```python
from build123d import *

# Parameters (mm, degrees)
CUT_EXTRUDE_1_DEPTH = 3
FILLET_1_R          = 0.3
CHAMFER_1_SIZE      = 1


with BuildPart() as part:
    # Эскиз1 → Повернуть1 (revolve)
    with BuildSketch(Plane.XY, mode=Mode.PRIVATE) as revolve_1_sk:
        Polygon((0, 0), (0, 5.9), (0.5, 5.9), (4, 3), (16, 3), (16, 0), align=None)
    revolve(revolve_1_sk.sketch.rotate(Axis((0, 0, 0), (1, 0, 0)), 90), axis=Axis((0, 0, 0), (1, 0, 0)))  # turned: the seam where the file's is

    # Эскиз2 → Вырез-Вытянуть1 (cut)
    with BuildSketch(Plane.ZY):
        Polygon((1.154700538, 2), (-1.154700538, 2), (-2.309401077, 0), (-1.154700538, -2), (1.154700538, -2), (2.309401077, 0), align=None)
    extrude(amount=-CUT_EXTRUDE_1_DEPTH, mode=Mode.SUBTRACT)

    # Скругление1
    fillet_1_edges = [part.edges().sort_by_distance(p)[0] for p in [
        (0, 0, -5.9),
    ]]
    fillet(fillet_1_edges, radius=FILLET_1_R)

    # Фаска1
    chamfer_1_edges = [part.edges().sort_by_distance(p)[0] for p in [
        (16, 0, -3),
    ]]
    chamfer(chamfer_1_edges, length=CHAMFER_1_SIZE)


solid = part.part
```
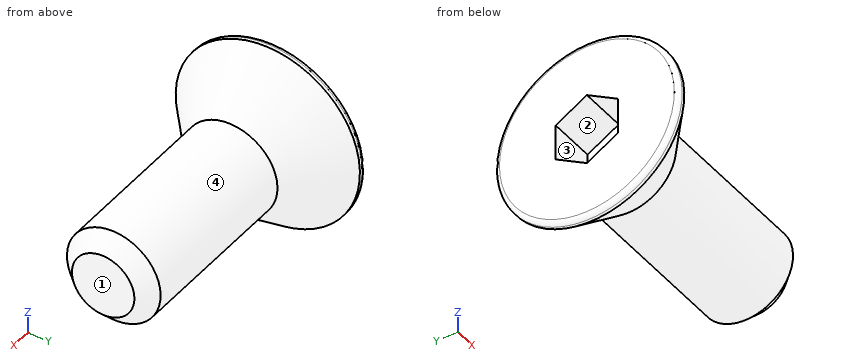
Read the model definition and answer for the solid it produces. Units are mm, in the model's axes. Face numbers are marked on the shaded views. Round coordinates to 2 decimals unless told otherwise and drop trailing zeros. Write each loop counter-clockwise with the first axis right and the second up, starting at its lowest first coordinate (ties: lowest second). Pieces come first, ordered by that corner, then holes. Notation, with made-up numbers: (38.25, 77.25) -> (58.25, 77.25) arc R26 cw to (58.25, 112.25) -> close; hole circle Ø3 at (73.5, -27.5). An arc over 180 degrees is marked (long way). Answer in a Markdown table with one row per item. Add a question column.
1) Find section A-A, the plane z = 0. Determine the outline of the cut face in (x, y).
2) Find section B-B, the plane x = 5. Determine the outline of the cut face in (y, z), and give its area (3 significant figures).
3) Given P1, Ø2.5, axis at x = 1.5, z = 0.5, coming from the +Y side; P2, Ø4, axis at x = 13.5, y = 4.5, coming from the +Z side; P3, Ø0.7, axis at x = 1.5, z = 0.5, coming from the -Y side; P4, Ø6, axis at x = 5, y = 1, coming from the +Z side, each flat-ended and moving along its own axis, determine where each tip first touches the part or whether it passes through.
4) Consider line 1 (Y direction, x = 12.75, z = 0); line 2 (X direction, y = 0.5, z = 1); line 3 (X direction, y = 1.5, z = 5.5). Determine where each line is inside the solid, lowest interval first.
5) Determine the mould class of the marked faces 1, 2, 3 and 4 for opening direction Y: pulls with the +Y half, pulls with the -Y half, needs draft (parallel to the pull), parting line crosses it, or undercut.
Findings below:
| question | item | result |
|---|---|---|
| 1 | outline | (0, -5.6) arc R0.3 ccw to (0.3, -5.9) -> (0.5, -5.9) -> (4, -3) -> (15, -3) -> (16, -2) -> (16, 2) -> (15, 3) -> (4, 3) -> (0.5, 5.9) -> (0.3, 5.9) arc R0.3 ccw to (0, 5.6) -> (0, 2) -> (3, 2) -> (3, -2) -> (0, -2) -> close |
| 2 | outline | circle Ø6 at (0, 0) |
| 2 | area | 28.3 mm² |
| 3 | P1 | y = 5.9 |
| 3 | P2 | z = 1.66 |
| 3 | P3 | y = -5.34 |
| 3 | P4 | z = 4.6 |
| 4 | line 1 | -3 to 3 |
| 4 | line 2 | 3 to 16 |
| 4 | line 3 | 0.02 to 0.74 |
| 5 | face 1 | needs draft |
| 5 | face 2 | undercut |
| 5 | face 3 | undercut |
| 5 | face 4 | parting line crosses it |
